Geometry check sheet. Reference: drawing and pictorial views, mm from the part's lowest x, y, z. Round coordinates to 2 decimals unless told otherwise and drop trailing zeros. Order: outer loops, then holes, each group sorted by start corner. A loop starts at its lowest first (then second) coordinate and runs counter-clockwise, first axis right, second up.
Q1. Mould release check, pull along Z, two halves, no side actions. Record for the marked faces 1, 2 and 3: +Z half, -Z half, draft (parallel to the pull), parting line (faces both ways), or undercut.
Q2. Scan lines: probe 1 along Y at (x, z) = (1.25, 0.2) (1 decimal); probe 2 along Z at (x, y) = (1.1, 7); probe 3 along Y at (x, z) = (0.4, 1.7) (1 decimal). Record each from-to range of solid material in increasing order.
Q3. Depth check by flat-ended pin: P1, Ø0.5, axis at x = 1, y = 8, coming from the -Z side; P2, Ø0.7, axis at y = 2.5, z = 1.5, coming from the +X side; P3, Ø0.5, axis at y = 1, z = 1, coming from the -X side; P4, Ø1.5, axis at y = 5.5, z = 1, coming from the -X side. Enter the tip coordinate at first touch or a pass-through.
Q4. Cross-section at C-C on y = 5.25. Record the cut outline in (x, z) (1 decimal).
Q5. Cross-section at D-D on z = 0.8. Record the cut outline in (x, y) (1 decimal).
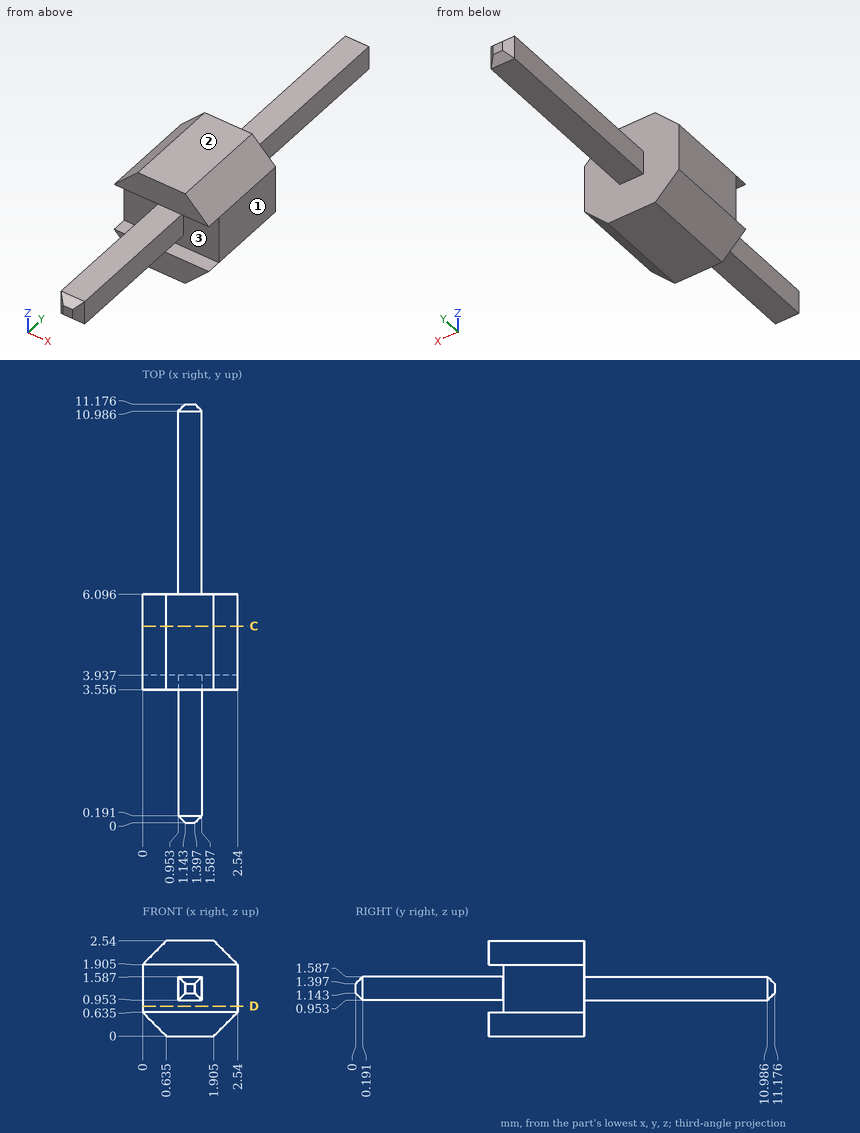
Results found:
1. face 1: draft
1. face 2: +Z half
1. face 3: undercut
2. probe 1: y = 3.6 to 6.1
2. probe 2: z = 0.95 to 1.59
2. probe 3: y = 3.9 to 6.1
3. P1: stops at z = 0.95
3. P2: stops at x = 1.59
3. P3: stops at x = 0.95
3. P4: stops at x = 0
4. outline: (0, 0.6) - (0.6, 0) - (1.9, 0) - (2.5, 0.6) - (2.5, 1.9) - (1.9, 2.5) - (0.6, 2.5) - (0, 1.9) - close
5. outline: (0, 3.9) - (2.5, 3.9) - (2.5, 6.1) - (0, 6.1) - close
